Print and shaded views of the part. All mm, measured from the part's lowest x, y and z. A direction names the side the tool comes from. Round coordinates to 2 decimals unless told otherwise and drop trailing zeros. Write each loop counter-clockwise with the first axis right and the second up, starting at its lowest first coordinate (ties: lowest second). Pieces come first, ordered by that corner, then holes.
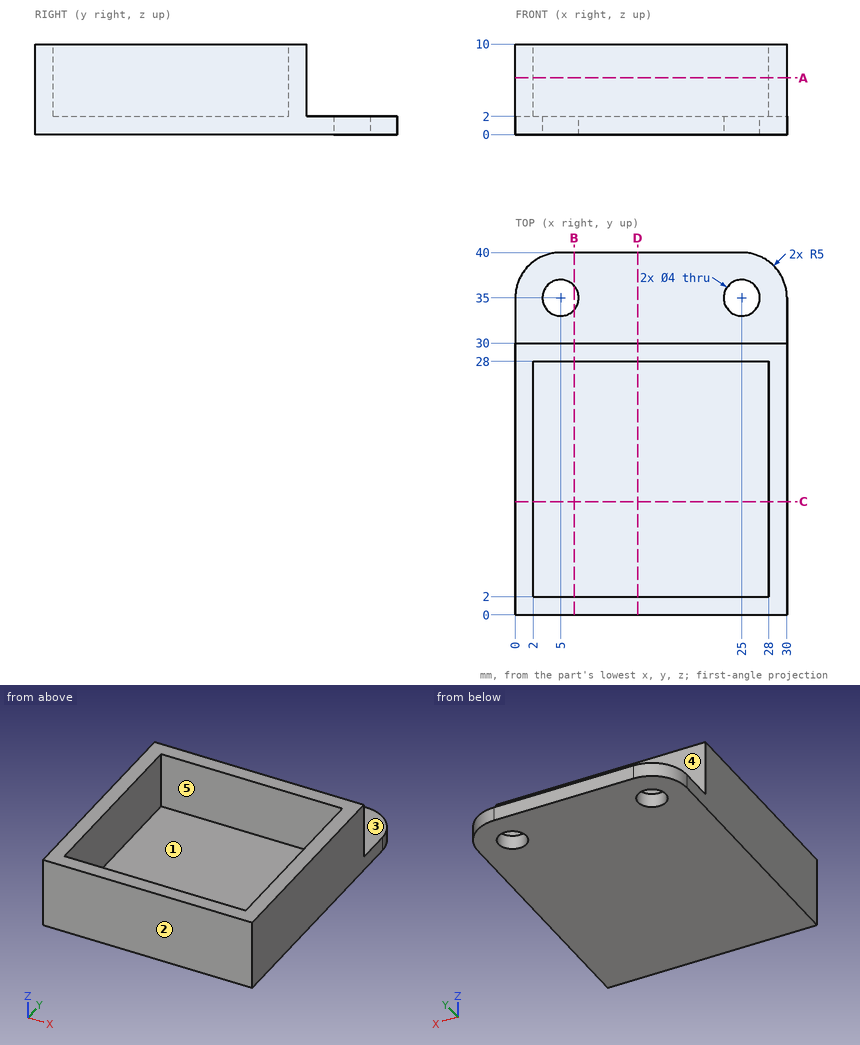
1) Slice it at A-A (z = 6.25). Write the cut outline in (x, y).
Results:
outline: (0, 0) - (30, 0) - (30, 30) - (0, 30) - close; hole (2, 2) - (28, 2) - (28, 28) - (2, 28) - close
2) Mould opens along Y. For the marked faces 3, 4 and 5 say: released by +Y, released by -Y, zero draft, split by the parting line, or undercut.
Results:
face 3: zero draft
face 4: released by +Y
face 5: undercut
3) Slice it at B-B (x = 6.5). Write the cut outline in (y, z).
Results:
outline: (0, 0) - (33.68, 0) - (33.68, 2) - (30, 2) - (30, 10) - (28, 10) - (28, 2) - (2, 2) - (2, 10) - (0, 10) - close; (36.32, 0) - (40, 0) - (40, 2) - (36.32, 2) - close
4) Wall check: L1, parallel to X at y = 19, z = 2.25; L2, parallel to Z at x = 22, y = 21. Give the ranges that are in metal, low to high.
Results:
L1: x = 0 to 2, 28 to 30
L2: z = 0 to 2
5) Slice it at C-C (y = 12.5). Write the cut outline in (x, z), plus the area to 3 significant figures.
Results:
outline: (0, 0) - (30, 0) - (30, 10) - (28, 10) - (28, 2) - (2, 2) - (2, 10) - (0, 10) - close
area: 92.0 mm2
6) Slice it at D-D (x = 13.5). Write the cut outline in (y, z), plus the area to 3 significant figures.
Results:
outline: (0, 0) - (40, 0) - (40, 2) - (30, 2) - (30, 10) - (28, 10) - (28, 2) - (2, 2) - (2, 10) - (0, 10) - close
area: 112 mm2
7) Which spindle directions (+Z, -Z, +X, -X, +Y, -Y) get a long thin tool onto all of the face, cutting with end or side? Do the marked faces 1 and 2. Say none if no direction does.
Results:
face 1: +Z
face 2: +Z, -Z, +X, -X, -Y
8) Pin check, flat tips, straight feed: pin 1 Ø1 at (x, z) = (8.5, 6.5) entering from +Y; pin 2 Ø8 at (x, y) = (11.5, 8.5) entering from +Z; pin 3 Ø2.5 at (x, y) = (5, 35) entering from -Z; pin 4 Ø1 at (x, z) = (4, 2) entering from +Y. Stop position of each tip, or through.
Results:
pin 1: stops at y = 30
pin 2: stops at z = 2
pin 3: passes through
pin 4: stops at y = 39.97
